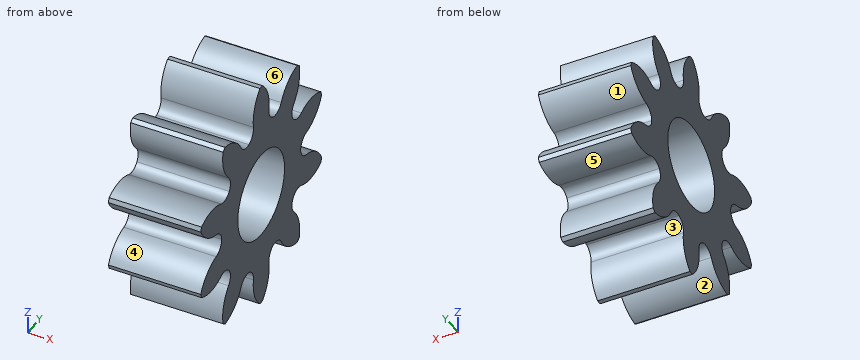
from build123d import *

# Parameters (mm, degrees)
BASPROSKE_W        = 10
BASPROSKE_H        = 6.75
TOOTHCUT_DEPTH     = 14.824796563
TEETHCUTS_COUNT    = 10
TEETHCUTS_ANGLE    = 324
BORSKE_R           = 2.5
BORE_DEPTH         = 50.0000508
SCALE1_SCALE       = 1.05
FILLET1_R          = 0.75
CUT_EXTRUDE1_START = -10.5
SKETCH1_R          = 10.265831804
CUT_EXTRUDE1_DEPTH = 5


with BuildPart() as part:
    # BasProSke → Base-Revolve (revolve)
    with BuildSketch(Plane(origin=(0, 0, 0), x_dir=(1, 0, 0), z_dir=(0, 1, 0)), mode=Mode.PRIVATE) as base_revolve_sk:
        with Locations((5, 3.375)):
            Rectangle(BASPROSKE_W, BASPROSKE_H)
    revolve(base_revolve_sk.sketch.rotate(Axis((-10, 0, 0), (1, 0, 0)), 180), axis=Axis((-10, 0, 0), (1, 0, 0)))

    # TooCutSke → ToothCut (cut, through all)
    with BuildSketch(Plane(origin=(0, 0, 0), x_dir=(0, 0, -1), z_dir=(1, 0, 0))):
        with BuildLine():
            ThreePointArc((0.665884296, 4.164854519), (0, 4.21775), (-0.665884296, 4.164854519))
            ThreePointArc((-0.665884296, 4.164854519), (-0.949936307, 5.537806691), (-1.991778305, 6.476022262))
            ThreePointArc((-1.991778305, 6.476022262), (0, 6.7754), (1.991778305, 6.476022262))
            ThreePointArc((1.991778305, 6.476022262), (0.949936307, 5.537806691), (0.665884296, 4.164854519))
        make_face()
    toothcut = extrude(amount=TOOTHCUT_DEPTH, mode=Mode.SUBTRACT)

    # TeethCuts: ToothCut ×10 about axis
    teethcuts_axis = Axis((-10, 0, 0), (1, 0, 0))
    for i in range(1, TEETHCUTS_COUNT):
        add(toothcut.rotate(teethcuts_axis, i * TEETHCUTS_ANGLE / (TEETHCUTS_COUNT - 1)), mode=Mode.SUBTRACT)

    # BorSke → Bore (cut, symmetric)
    with BuildSketch(Plane(origin=(0, 0, 0), x_dir=(0, 0, -1), z_dir=(1, 0, 0))):
        with Locations(Location((0, 0, 0), (0, 0, 180))):
            Circle(BORSKE_R)
    extrude(amount=BORE_DEPTH, both=True, mode=Mode.SUBTRACT)


with BuildPart() as part_1:
    # Scale1: scaled about (5, 0, 0)
    add(part.part.scale(SCALE1_SCALE).moved(Location((-0.25, 0, 0))))

    # Fillet1
    # the kernel refuses this fillet: 0.75 mm, written as the material it adds along each edge
    with BuildSketch(Plane(origin=(-0.25, 3.126943172, -3.136089365), x_dir=(0, 0.6486282387058202, 0.7611053855763902), z_dir=(1, 0, 0)), Plane(origin=(-0.25, 0.686403088, -4.375120673), x_dir=(0, 0.9721177892266772, 0.23449307850987308), z_dir=(1, 0, 0)), Plane(origin=(-0.25, -2.016319645, -3.94300459), x_dir=(0, 0.9242913853313495, -0.38168761442081794), z_dir=(1, 0, 0)), Plane(origin=(-0.25, -3.948876807, -2.004794771), x_dir=(0, 0.5234170877481713, -0.8520766117276212), z_dir=(1, 0, 0)), Plane(origin=(-0.25, -4.373097245, 0.69917851), x_dir=(0, -0.07738474706232469, -0.9970013043733192), z_dir=(1, 0, 0))) as fillet1_piece_1:
        with BuildLine():
            CenterArc((0.778083465, -0.747536247), FILLET1_R, 94.645414963, 79.810658705)
            ThreePointArc((0.031591647, -0.675079607), (0.040059779, -0.336404325), (0, 0))
            ThreePointArc((0, 0), (0.358670863, -0.01454809), (0.717341725, 0))
        make_face()
    extrude(amount=10.5)
    with BuildSketch(Plane(origin=(-0.25, 3.948876807, -2.004794771), x_dir=(0, 0.8266776070022068, -0.562675869467587), z_dir=(1, 0, 0)), Plane(origin=(-0.25, 2.016319645, -3.94300459), x_dir=(0, 0.3380636550401047, -0.9411232465203083), z_dir=(1, 0, 0)), Plane(origin=(-0.25, -0.686403088, -4.375120673), x_dir=(0, -0.27967912278629736, -0.9600935310049158), z_dir=(1, 0, 0)), Plane(origin=(-0.25, -3.126943172, -3.136089365), x_dir=(0, -0.7905939816520889, -0.6123407190245448), z_dir=(1, 0, 0)), Plane(origin=(-0.25, -4.373097245, -0.69917851), x_dir=(0, -0.9995288108278918, -0.030694565072345244), z_dir=(1, 0, 0))) as fillet1_piece_2:
        with BuildLine():
            CenterArc((0.78309116, -0.742288727), FILLET1_R, 98.223237645, 79.810658705)
            ThreePointArc((0.033532686, -0.716557541), (0.031298529, -0.357598709), (0, 0))
            ThreePointArc((0, 0), (0.337909199, -0.024290509), (0.675818399, 0))
        make_face()
    extrude(amount=10.5)
    with BuildSketch(Plane(origin=(-0.25, -3.948876807, 2.004794771), x_dir=(0, 0.5234170877481569, 0.8520766117276299), z_dir=(1, 0, 0)), Plane(origin=(-0.25, -2.016319645, 3.94300459), x_dir=(0, 0.9242913853313433, 0.38168761442083243), z_dir=(1, 0, 0)), Plane(origin=(-0.25, 0.686403088, 4.375120673), x_dir=(0, 0.9721177892266811, -0.23449307850985693), z_dir=(1, 0, 0)), Plane(origin=(-0.25, 3.126943172, 3.136089365), x_dir=(0, 0.6486282387058309, -0.761105385576381), z_dir=(1, 0, 0)), Plane(origin=(-0.25, 4.373097245, 0.69917851), x_dir=(0, 0.07738474706233216, -0.9970013043733188), z_dir=(1, 0, 0))) as fillet1_piece_3:
        with BuildLine():
            CenterArc((0.778083465, 0.747536247), FILLET1_R, 185.543926332, 79.810658705)
            ThreePointArc((0.031591647, 0.675079607), (0.040059779, 0.336404325), (0, 0))
            ThreePointArc((0, 0), (0.358670863, 0.01454809), (0.717341725, 0))
        make_face()
    extrude(amount=10.5)
    with BuildSketch(Plane(origin=(-0.25, -3.126943172, 3.136089365), x_dir=(0, -0.7905939816520986, 0.6123407190245325), z_dir=(1, 0, 0)), Plane(origin=(-0.25, -0.686403088, 4.375120673), x_dir=(0, -0.2796791227863126, 0.9600935310049113), z_dir=(1, 0, 0)), Plane(origin=(-0.25, 2.016319645, 3.94300459), x_dir=(0, 0.33806365504009167, 0.9411232465203131), z_dir=(1, 0, 0)), Plane(origin=(-0.25, 3.948876807, 2.004794771), x_dir=(0, 0.826677607002198, 0.5626758694676001), z_dir=(1, 0, 0)), Plane(origin=(-0.25, 4.373097245, -0.69917851), x_dir=(0, 0.9995288108278919, -0.030694565072338184), z_dir=(1, 0, 0))) as fillet1_piece_4:
        with BuildLine():
            CenterArc((0.78309116, 0.742288727), FILLET1_R, 181.96610365, 79.810658705)
            ThreePointArc((0.033532686, 0.716557541), (0.031298529, 0.357598709), (0, 0))
            ThreePointArc((0, 0), (0.337909199, 0.024290509), (0.675818399, 0))
        make_face()
    extrude(amount=10.5)

    # Sketch1 → Cut-Extrude1 (cut)
    with BuildSketch(Plane(origin=(10.25, 0, 0), x_dir=(0, 0, -1), z_dir=(1, 0, 0)).offset(CUT_EXTRUDE1_START)):
        Circle(SKETCH1_R)
    extrude(amount=CUT_EXTRUDE1_DEPTH, mode=Mode.SUBTRACT)


solid = part_1.part
Could you check a few things on this model? Use its own coordinates, in mm. Face numbers are marked on the shaded views. A direction names the side the tool comes from. Round coordinates to 2 decimals unless told otherwise and drop trailing zeros. Order: outer loops, then holes, each group sorted by start corner. A loop starts at its lowest first (then second) coordinate and runs counter-clockwise, first axis right, second up. Notation, with made-up numbers: M 82,-5 L 86,-5 A22 ccw 86,32 Z; hole C 33,-35 d5. An arc over 180 degrees is marked long. One line per item, written item: value.
(1) Which directions (+Z, -Z, +X, -X, +Y, -Y) give clear straight access to the entire face, cutting with the end or side of a thin tool? Please do the marked faces 1, 2 and 3.
Ans:
face 1: +X, -X, +Y
face 2: -Z, +X, -X
face 3: +X, -X
(2) Imagine slicing it at A-A (y = 4.75). Write out the boundary of the cut face in (x, z).
Ans:
outline: M 4.75,-2.49 L 10.25,-2.49 L 10.25,-0.6 L 4.75,-0.6 Z; M 4.75,0.6 L 10.25,0.6 L 10.25,2.49 L 4.75,2.49 Z
(3) Imagine slicing it at B-B (z = -5.25). Write out the boundary of the cut face in (x, y).
Ans:
outline: M 4.75,-4.32 L 10.25,-4.32 L 10.25,-2.78 L 4.75,-2.78 Z; M 4.75,-0.9 L 10.25,-0.9 L 10.25,0.9 L 4.75,0.9 Z; M 4.75,2.78 L 10.25,2.78 L 10.25,4.32 L 4.75,4.32 Z
(4) I need wall thicknesses on line 1 along Y through (x, z) = (7.9, 4.75); line 2 along Y through (x, z) = (9.3, 5); line 3 along Y through (x, z) = (7.45, 1.75). Which ranges of each line are inside material? Lowest first, please. Write a range as from..to.
Ans:
line 1: y = -4.28..-2.35, -0.89..0.89, 2.35..4.28
line 2: y = -4.32..-2.53, -0.87..0.87, 2.53..4.32
line 3: y = -6.61..-1.96, 1.96..6.61
(5) I'm going to push flat-ended pins straight in: P1, Ø2, axis at x = 7.5, z = 4, coming from the +Y side; P2, Ø1, axis at x = 8, z = 0.5, coming from the +Y side; P3, Ø3, axis at y = 0, z = 0, coming from the +X side. Where does each tip first touch, or does it pass through?
Ans:
P1: stops at y = 4.32
P2: stops at y = 5.82
P3: passes through
(6) If we mould it in two halves opening along Z, with no side actions, what happens to the marked faces 4, 5 and 6? For each: released by +Z, released by -Z, zero draft, split by the parting line, or undercut.
Ans:
face 4: undercut
face 5: released by -Z
face 6: released by +Z
